Autodesk Inventor part; units mm, degrees
ref_plane "YZ Plane" through (0, 0, 0) normal (1, 0, 0) x (0, 1, 0)
ref_plane "XZ Plane" through (0, 0, 0) normal (0, 1, 0) x (-1, 0, 0)
ref_plane "XY Plane" through (0, 0, 0) normal (0, 0, 1) x (1, 0, 0)
sketch "スケッチ1" plane through (0, 0, 0) normal (1, 0, 0) x (0, 1, 0)
  line L0 (-7.5, 0) -> (7.5, 0)
  line L1 (0, 0) -> (0, 4.0415) construction
  line L2 (-7.1874, 4.0415) -> (-7.5, 3.5)
  line L3 (-7.5, 3.5) -> (-7.5, 0)
  line L4 (-7.1874, 4.0415) -> (7.1874, 4.0415)
  line L5 (7.1874, 4.0415) -> (7.5, 3.5)
  line L6 (7.5, 3.5) -> (7.5, 0)
  line L7 (-7.5, 2) -> (-14.2, 2)
  line L8 (-14.5, 1.7) -> (-14.5, 0)
  line L9 (-14.5, 0) -> (-7.5, 0)
  line L10 (-14.2, 2) -> (-14.5, 1.7)
  point P0 (7.5, 1.5)
  point P1 (-14.5, 2)
  dimension "d1" = 3.5
  dimension "d2" = 4.0415
  dimension "d3" = 30
  dimension "d4" = 15
  dimension "d18" = 7
  dimension "d19" = 4
  dimension "d22" = 0.3
  dimension "d23" = 0.3
revolve "回転1" add sketch "スケッチ1" angle 360 about axis through (0, -7.5, 0) along (0, 1, 0)
sketch "スケッチ2" plane through (0, 7.5, 0) normal (0, 1, 0) x (1, 0, 0)
  line L0 (0, -4.0415) -> (-3.5, -2.0207)
  line L1 (-3.5, -2.0207) -> (-3.5, 2.0207)
  line L2 (-3.5, 2.0207) -> (0, 4.0415)
  line L3 (0, 4.0415) -> (3.5, 2.0207)
  line L4 (3.5, 2.0207) -> (3.5, -2.0207)
  line L5 (3.5, -2.0207) -> (0, -4.0415)
  circle A0 centre (0, 0) radius 4.0415
  point P0 (0, 0)
  point P1 (0, 0)
  point P2 (3.5, 2.0207)
  point P3 (3.5, 2.0207)
  point P4 (0, 4.0415)
  point P5 (0, 4.0415)
  point P6 (-3.5, 2.0207)
  point P7 (-3.5, 2.0207)
  point P8 (-3.5, -2.0207)
  point P9 (3.5, -2.0207)
  point P10 (3.5, -2.0207)
extrude "押し出し1" cut sketch "スケッチ2" against normal through all contours A0 L0 | L5 A0 | A0 L1 | L4 A0 | A0 L2 | L3 A0
hole "穴1" at (0, 7.5, 0) direction (0, -1, 0) diameter 3.242 depth 8 tip angle 118 countersink diameter 4 countersink angle 90
thread "ねじ1"
equation "\"d2\" = 1.1547 * d1"
properties part number "BSL-415BE" material "アルミニウム 2014-T4"
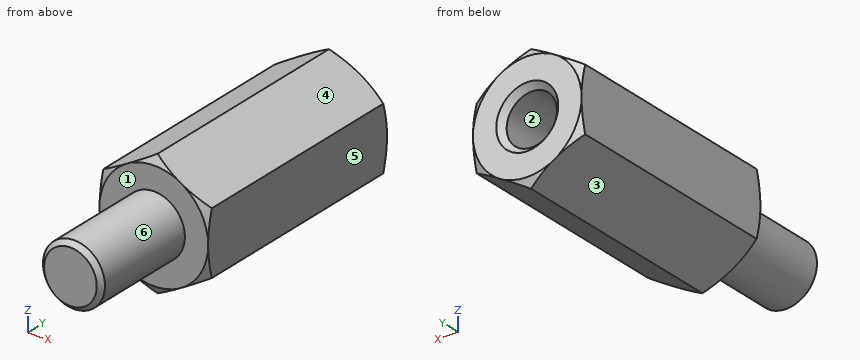
For this review, take the finished solid that the model builds, in its own axes (mm). Face numbers are marked on the shaded views. A direction names the side the tool comes from. Round coordinates to 2 decimals unless told otherwise and drop trailing zeros. Write each loop counter-clockwise with the first axis right and the second up, starting at its lowest first coordinate (ties: lowest second). Pieces come first, ordered by that corner, then holes.
1) Mouldability with a two-part tool opening along X and no side actions: class the marked faces 1, 2, 3 and 4 as +X half, -X half, draft (parallel to the pull), parting line (faces both ways), or undercut.
Answer below:
face 1: draft
face 2: undercut
face 3: -X half
face 4: +X half
2) Take a section at B-B on y = -4. Give the boundary of the cut face in (x, z), then the cut area to 3 significant figures.
Answer below:
outline: (-3.5, -2.02) - (0, -4.04) - (3.5, -2.02) - (3.5, 2.02) - (0, 4.04) - (-3.5, 2.02) - close
area: 42.4 mm2
3) For line 1 along X through (y, z) = (2.5, 0); line 2 along Y through (x, z) = (-3, 1.5); line 3 along Z through (x, y) = (-0.75, 3.5), list the stretches that pass through material, from the lowest coordinate up.
Answer below:
line 1: x = -3.5 to -1.62, 1.62 to 3.5
line 2: y = -7.5 to 7.5
line 3: z = -3.61 to -1.44, 1.44 to 3.61
4) Take a section at A-A on y = 3.25. Give the boundary of the cut face in (x, z).
Answer below:
outline: (-3.5, -2.02) - (0, -4.04) - (3.5, -2.02) - (3.5, 2.02) - (0, 4.04) - (-3.5, 2.02) - close; hole circle Ø3.24 at (0, 0)
5) Take a section at C-C on y = -12.25. Give the boundary of the cut face in (x, z).
Answer below:
outline: circle Ø4 at (0, 0)
6) Insertion check: pin 1 Ø4 at (y, z) = (-10.5, -2) entering from +X; pin 2 Ø4 at (x, y) = (2.5, 4.5) entering from -Z; pin 3 Ø1.9 at (x, z) = (0, 0) entering from +Y. Each pin has a flat end and moves straight along its axis. Give the tip position at first contact, or say it passes through.
Answer below:
pin 1: stops at x = 2
pin 2: stops at z = -3.75
pin 3: stops at y = -0.9
7) Machinability: for the marked faces 5 and 6, which of the approach directions +Z, -Z, +X, -X, +Y, -Y give a long, thin tool a straight path to every point of the face, cutting with its end or side? Answer none if there is none.
Answer below:
face 5: +Z, -Z, +X, +Y, -Y
face 6: -Y
